Geometry: final body of the model. Coordinates: model frame, mm. A direction names the side the tool comes from. Give positions to 0.01 mm unless a question says otherwise; leave off trailing zeros. Write each loop counter-clockwise with the first axis right and the second up, starting at its lowest first coordinate (ties: lowest second). Pieces come first, ordered by that corner, then holes. Notation, with made-up numbers: M -37,-23.5 L 20,-23.5 A27 cw 20,-5.5 Z; hole C -33,42 d1. An arc over 180 degrees is marked long. Answer as a JSON object with one key per item and string values.
from build123d import *

# Parameters (mm, degrees)
SKETCH1_W                                     = 82
SKETCH1_H                                     = 323.5
BASE_EXTRUSION_DEPTH                          = 2
ACCESS_PORTS_DEPTH                            = 167.877387623
SKETCH4_W                                     = 82
SKETCH4_H                                     = 323.5
SKETCH4_W_2                                   = 78
SKETCH4_H_2                                   = 319.5
CORNER_RAIL_MOUNTS_DEPTH                      = 7
M3X0_5_TAPPED_HOLE_FOR_END_D                  = 2.5
M3X0_5_TAPPED_HOLE_FOR_END_DEPTH              = 2
SKETCH14_W                                    = 9
SKETCH14_H                                    = 32
ANTENNA_CUTOUT_DEPTH                          = 2
SKETCH15_W                                    = 2
SKETCH15_H                                    = 2
SLITS_IN_CORNERS_DEPTH                        = 7
M3X0_5_TAPPED_HOLES_FOR_RAILS_D               = 2.5
M3X0_5_TAPPED_HOLES_FOR_RAILS_DEPTH           = 2
M3X0_5_TAPPED_HOLES_FOR_RAILS_ON_FACE_2_D     = 2.5
M3X0_5_TAPPED_HOLES_FOR_RAILS_ON_FACE_2_DEPTH = 2
SKETCH17_W                                    = 2
SKETCH17_H                                    = 100
SKETCH17_W_2                                  = 1
SUPPORT_FOR_PAYLOAD_DEPTH                     = 1


with BuildPart() as part:
    # Sketch1 → Base Extrusion (new body)
    with BuildSketch(Plane(origin=(0, 0, 0), x_dir=(0, 0, -1), z_dir=(1, 0, 0))):
        Rectangle(SKETCH1_W, SKETCH1_H)
    extrude(amount=BASE_EXTRUSION_DEPTH)

    # Sketch8 → Access Ports (cut, through all)
    with BuildSketch(Plane(origin=(2, 0, 0), x_dir=(0, 0, -1), z_dir=(1, 0, 0))):
        with BuildLine():
            Line((-30.5, 55.75), (30.5, 55.75))
            ThreePointArc((30.5, 55.75), (31.914213562, 56.335786438), (32.5, 57.75))
            Line((32.5, 57.75), (32.5, 139.25))
            ThreePointArc((32.5, 139.25), (31.914213562, 140.664213562), (30.5, 141.25))
            Line((30.5, 141.25), (-30.5, 141.25))
            ThreePointArc((-30.5, 141.25), (-31.914213562, 140.664213562), (-32.5, 139.25))
            Line((-32.5, 139.25), (-32.5, 57.75))
            ThreePointArc((-32.5, 57.75), (-31.914213562, 56.335786438), (-30.5, 55.75))
        make_face()
        with BuildLine():
            Line((-30.5, -56.75), (30.5, -56.75))
            ThreePointArc((30.5, -56.75), (31.914213562, -56.164213562), (32.5, -54.75))
            Line((32.5, -54.75), (32.5, 26.75))
            ThreePointArc((32.5, 26.75), (31.914213562, 28.164213562), (30.5, 28.75))
            Line((30.5, 28.75), (-30.5, 28.75))
            ThreePointArc((-30.5, 28.75), (-31.914213562, 28.164213562), (-32.5, 26.75))
            Line((-32.5, 26.75), (-32.5, -54.75))
            ThreePointArc((-32.5, -54.75), (-31.914213562, -56.164213562), (-30.5, -56.75))
        make_face()
        with BuildLine():
            Line((-32.5, -159.75), (32.5, -159.75))
            Line((32.5, -159.75), (32.5, -85.75))
            ThreePointArc((32.5, -85.75), (31.914213562, -84.335786438), (30.5, -83.75))
            Line((30.5, -83.75), (-30.5, -83.75))
            ThreePointArc((-30.5, -83.75), (-31.914213562, -84.335786438), (-32.5, -85.75))
            Line((-32.5, -85.75), (-32.5, -159.75))
        make_face()
    extrude(amount=-ACCESS_PORTS_DEPTH, mode=Mode.SUBTRACT)

    # Sketch4 → Corner Rail Mounts (add)
    with BuildSketch(Plane(origin=(2, 0, 0), x_dir=(0, 0, -1), z_dir=(1, 0, 0))):
        Rectangle(SKETCH4_W, SKETCH4_H)
        Rectangle(SKETCH4_W_2, SKETCH4_H_2, mode=Mode.SUBTRACT)
    extrude(amount=CORNER_RAIL_MOUNTS_DEPTH)

    # M3x0.5 Tapped Hole For End
    with Locations(Plane.XZ.offset(161.75)):
        with Locations((5.5, 0)):
            Hole(M3X0_5_TAPPED_HOLE_FOR_END_D / 2, depth=M3X0_5_TAPPED_HOLE_FOR_END_DEPTH)

    # Sketch14 → Antenna Cutout (cut)
    with BuildSketch(Plane(origin=(0, 161.75, 0), x_dir=(1, 0, 0), z_dir=(0, 1, 0))):
        with Locations((4.5, 0)):
            Rectangle(SKETCH14_W, SKETCH14_H)
    extrude(amount=-ANTENNA_CUTOUT_DEPTH, mode=Mode.SUBTRACT)

    # Sketch15 → Slits In Corners (cut)
    with BuildSketch(Plane(origin=(9, 0, 0), x_dir=(0, 0, -1), z_dir=(1, 0, 0))):
        with Locations((-40, -158.75)):
            Rectangle(SKETCH15_W, SKETCH15_H)
        with Locations((40, -158.75)):
            Rectangle(SKETCH15_W, SKETCH15_H)
        with Locations((40, 158.75)):
            Rectangle(SKETCH15_W, SKETCH15_H)
        with Locations((-40, 158.75)):
            Rectangle(SKETCH15_W, SKETCH15_H)
    extrude(amount=-SLITS_IN_CORNERS_DEPTH, mode=Mode.SUBTRACT)

    # M3x0.5 Tapped Holes For Rails
    with Locations(Plane(origin=(4.5, 136.75, -41), x_dir=(-1, 0, 0), z_dir=(0, 0, -1))):
        with Locations((0, 0), (0, -91.166666667), (0, -182.333333333), (0, -273.5)):
            Hole(M3X0_5_TAPPED_HOLES_FOR_RAILS_D / 2, depth=M3X0_5_TAPPED_HOLES_FOR_RAILS_DEPTH)

    # M3x0.5 Tapped Holes For Rails on face 2
    with Locations(Plane(origin=(4.5, 111.75, 41), x_dir=(1, 0, 0), z_dir=(0, 0, 1))):
        with Locations((0, 0), (0, -111.75), (0, -223.5)):
            Hole(M3X0_5_TAPPED_HOLES_FOR_RAILS_ON_FACE_2_D / 2, depth=M3X0_5_TAPPED_HOLES_FOR_RAILS_ON_FACE_2_DEPTH)

    # Sketch17 → Support For Payload (add)
    with BuildSketch(Plane(origin=(9, 0, 0), x_dir=(0, 0, -1), z_dir=(1, 0, 0))):
        with Locations((40, 107.75)):
            Rectangle(SKETCH17_W, SKETCH17_H)
        with Locations((-39.5, 107.75)):
            Rectangle(SKETCH17_W_2, SKETCH17_H)
    extrude(amount=SUPPORT_FOR_PAYLOAD_DEPTH)


solid = part.part
1) Set-up query: faces 1 (the flat face through (4, -2, 41)), 2 (the flat face through (6, 159.75, -28)), 3 (the flat face through (4, -159.75, 1)). Return all of +Z, -Z, +X, -X, +Y, -Y with unobstructed straight access to the full face (end or side cutting, diameter ignored); none if empty.
Geometry check:
{"face 1": "+Z, +X, -X, +Y, -Y", "face 2": "+Z, -Z, +X", "face 3": "+X"}
2) Contact query for flat-ended pins moving along their axis: P1, Ø5, axis at y = -52, z = -0.5, coming from the +X side; P2, Ø2, axis at x = 1, z = 1.5, coming from the +Y side; P3, Ø3, axis at x = 4.5, y = 136.75, coming from the -Z side; P4, Ø0.8, axis at x = 9.5, y = 125.5, coming from the +Z side. Output: stop coordinate, or through.
Geometry check:
{"P1": "passes through", "P2": "stops at y = 159.75", "P3": "stops at z = -41", "P4": "stops at z = 40"}
3) Cut plane C-C on y = 121. Return loops of the section in (x, z), and give its area (3 significant figures).
Geometry check:
{"outline": "M 0,-41 L 10,-41 L 10,-39 L 2,-39 L 2,-32.5 L 0,-32.5 Z; M 0,32.5 L 2,32.5 L 2,39 L 10,39 L 10,40 L 9,40 L 9,41 L 0,41 Z", "area": "65.0 mm2"}
4) Cut plane A-A on y = -101. Return loops of the section in (x, z).
Geometry check:
{"outline": "M 0,-41 L 9,-41 L 9,-39 L 2,-39 L 2,-32.5 L 0,-32.5 Z; M 0,32.5 L 2,32.5 L 2,39 L 9,39 L 9,41 L 0,41 Z"}
5) Pull-direction query (Y, two-part tool) for faces 4 (the flat face through (6, -2, -39)), 5 (the flat face through (5, -2, -41)), 6 (the flat face through (3, -161.75, 1)), 7 (the flat face through (4, 161.75, -28)); classes: pulls with the +Y half, pulls with the -Y half, needs draft (parallel to the pull), parting line crosses it, or undercut.
Geometry check:
{"face 4": "undercut", "face 5": "needs draft", "face 6": "pulls with the -Y half", "face 7": "pulls with the +Y half"}
6) Line query: line 1 (Y direction, x = 4.5, z = 39.65); line 2 (Z direction, x = 4.75, y = -16.5); line 3 (Y direction, x = 5.5, z = -24.5). Output: solid intervals per line, ascending. Write a range as from..to.
Geometry check:
{"line 1": "y = -161.75..-159.75, -157.75..-113, -110.5..-1.25, 1.25..110.5, 113..157.75, 159.75..161.75", "line 2": "z = -41..-39, 39..41", "line 3": "y = -161.75..-159.75, 159.75..161.75"}
7) Cut plane B-B on z = -25. Return loops of the section in (x, y).
Geometry check:
{"outline": "M 0,-161.75 L 9,-161.75 L 9,-159.75 L 0,-159.75 Z; M 0,-83.75 L 2,-83.75 L 2,-56.75 L 0,-56.75 Z; M 0,28.75 L 2,28.75 L 2,55.75 L 0,55.75 Z; M 0,141.25 L 2,141.25 L 2,159.75 L 9,159.75 L 9,161.75 L 0,161.75 Z"}
